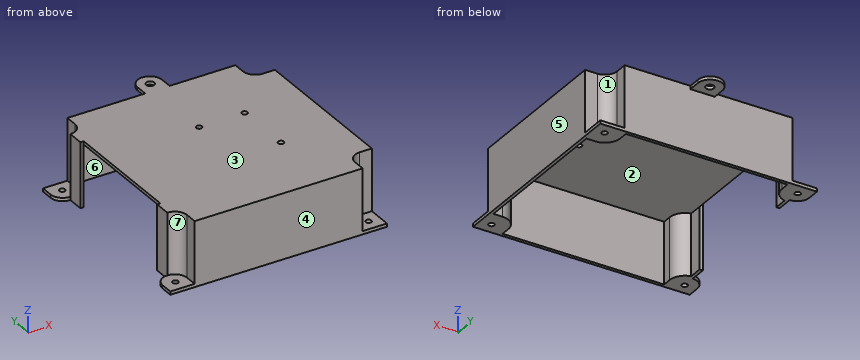
```python
from build123d import *

# Parameters (mm, degrees)
ESQUISSE1_W                = 126
ESQUISSE1_H                = 126
BOSS_EXTRU_1_DEPTH         = 40
ENL_V_MAT_EXTRU_1_DEPTH    = 38
ENL_V_MAT_EXTRU_2_REACH    = 223.428
ESQUISSE4_R                = 1.75
ENL_V_MAT_EXTRU_5_DEPTH    = 38
COQUE1_DEPTH               = 38
BOSS_EXTRU_3_DEPTH         = 2
ENL_V_MAT_EXTRU_6_REACH    = 228.624
ESQUISSE13_R               = 1.75
ENL_V_MAT_EXTRU_7_REACH    = 228.968
ESQUISSE14_R               = 1.75
R_P_TITION_LIN_AIRE1_COUNT = 2
R_P_TITION_LIN_AIRE1_PITCH = 28
ENL_V_MAT_EXTRU_8_REACH    = 228.968
ESQUISSE15_R               = 1.75
ESQUISSE16_W               = 40
ESQUISSE16_H               = 76
ENL_V_MAT_EXTRU_9_DEPTH    = 2
BOSS_EXTRU_4_DEPTH         = 2
ENL_V_MAT_EXTRU_10_REACH   = 239.591
ESQUISSE19_R               = 2.5


# Read off the part's stored shape, not the designer's step: Coque1
with BuildPart() as part:
    # Esquisse1 → Boss.-Extru.1 (new body)
    with BuildSketch(Plane.XY):
        with Locations((-88.440384558, 94.010362694)):
            Rectangle(ESQUISSE1_W, ESQUISSE1_H)
    extrude(amount=BOSS_EXTRU_1_DEPTH)

    # Esquisse2 → Enlèv. mat.-Extru.1 (cut)
    with BuildSketch(Plane.XY.offset(40)):
        with BuildLine():
            Line((-40.440384558, 31.010362694), (-25.440384558, 31.010362694))
            Line((-25.440384558, 31.010362694), (-25.440384558, 46.010362694))
            Line((-25.440384558, 46.010362694), (-32.940384558, 46.010362694))
            ThreePointArc((-32.940384558, 46.010362694), (-38.243685417, 43.813663553), (-40.440384558, 38.510362694))
            Line((-40.440384558, 38.510362694), (-40.440384558, 31.010362694))
        make_face()
    enl_v_mat_extru_1 = extrude(amount=-ENL_V_MAT_EXTRU_1_DEPTH, mode=Mode.SUBTRACT)

    # Esquisse4 → Enlèv. mat.-Extru.2 (cut, up to next)
    with BuildSketch(Plane.XY.offset(2), mode=Mode.PRIVATE) as enl_v_mat_extru_2_sk1:
        with Locations((-32.440384558, 38.010362694)):
            Circle(ESQUISSE4_R)
    enl_v_mat_extru_2_tool1 = extrude(enl_v_mat_extru_2_sk1.sketch, amount=-ENL_V_MAT_EXTRU_2_REACH, mode=Mode.PRIVATE) & part.part
    enl_v_mat_extru_2 = enl_v_mat_extru_2_tool1.solids().sort_by_distance((-32.440385, 38.010363, 2))[0]
    add(enl_v_mat_extru_2, mode=Mode.SUBTRACT)

    # Symétrie1: Enlèv. mat.-Extru.1, Enlèv. mat.-Extru.2 across plane
    add(enl_v_mat_extru_1.mirror(Plane(origin=(0, 94.010362694, 0), x_dir=(0, 0, 1), z_dir=(0, -1, 0))), mode=Mode.SUBTRACT)
    add(enl_v_mat_extru_2.mirror(Plane(origin=(0, 94.010362694, 0), x_dir=(0, 0, 1), z_dir=(0, -1, 0))), mode=Mode.SUBTRACT)

    # Esquisse10 → Enlèv. mat.-Extru.5 (cut)
    with BuildSketch(Plane.XY.offset(40)):
        with BuildLine():
            Line((-151.440384558, 46.010362694), (-151.440384558, 31.010362694))
            Line((-151.440384558, 31.010362694), (-143.940384558, 31.010362694))
            Line((-143.940384558, 31.010362694), (-143.940384558, 38.510362694))
            ThreePointArc((-143.940384558, 38.510362694), (-146.137083699, 43.813663553), (-151.440384558, 46.010362694))
        make_face()
    enl_v_mat_extru_5 = extrude(amount=-ENL_V_MAT_EXTRU_5_DEPTH, mode=Mode.SUBTRACT)

    # Symétrie3: Enlèv. mat.-Extru.5 across plane
    add(enl_v_mat_extru_5.mirror(Plane(origin=(0, 94.010362694, 0), x_dir=(0, 0, 1), z_dir=(0, -1, 0))), mode=Mode.SUBTRACT)

    # Coque1 outline → Coque1 (cut)
    with BuildSketch(Plane.XY):
        with BuildLine():
            Line((-42.440384558, 155.010362694), (-141.940384558, 155.010362694))
            Line((-141.940384558, 155.010362694), (-141.940384558, 149.510362694))
            ThreePointArc((-141.940384558, 149.510362694), (-144.049511808, 143.541694501), (-149.440384558, 140.223274884))
            Line((-149.440384558, 140.223274884), (-149.440384558, 47.797450505))
            ThreePointArc((-149.440384558, 47.797450505), (-144.049511808, 44.479030887), (-141.940384558, 38.510362694))
            Line((-141.940384558, 38.510362694), (-141.940384558, 33.010362694))
            Line((-141.940384558, 33.010362694), (-42.440384558, 33.010362694))
            Line((-42.440384558, 33.010362694), (-42.440384558, 38.510362694))
            ThreePointArc((-42.440384558, 38.510362694), (-39.657898979, 45.227877116), (-32.940384558, 48.010362694))
            Line((-32.940384558, 48.010362694), (-27.440384558, 48.010362694))
            Line((-27.440384558, 48.010362694), (-27.440384558, 140.010362694))
            Line((-27.440384558, 140.010362694), (-32.940384558, 140.010362694))
            ThreePointArc((-32.940384558, 140.010362694), (-39.657898979, 142.792848273), (-42.440384558, 149.510362694))
            Line((-42.440384558, 149.510362694), (-42.440384558, 155.010362694))
        make_face()
    extrude(amount=COQUE1_DEPTH, mode=Mode.SUBTRACT)

    # Esquisse12 → Boss.-Extru.3 (add)
    with BuildSketch(Plane.XY.offset(2)):
        with BuildLine():
            Line((-158.940384558, 31.010362694), (-158.940384558, 38.510362694))
            ThreePointArc((-158.940384558, 38.510362694), (-156.743685417, 43.813663553), (-151.440384558, 46.010362694))
            Line((-151.440384558, 46.010362694), (-151.440384558, 31.010362694))
            Line((-151.440384558, 31.010362694), (-158.940384558, 31.010362694))
        make_face()
    boss_extru_3 = extrude(amount=-BOSS_EXTRU_3_DEPTH)

    # Esquisse13 → Enlèv. mat.-Extru.6 (cut, up to next)
    with BuildSketch(Plane.XY.offset(2), mode=Mode.PRIVATE) as enl_v_mat_extru_6_sk1:
        with Locations((-151.440384558, 38.010362694)):
            Circle(ESQUISSE13_R)
    enl_v_mat_extru_6_tool1 = extrude(enl_v_mat_extru_6_sk1.sketch, amount=-ENL_V_MAT_EXTRU_6_REACH, mode=Mode.PRIVATE) & part.part
    enl_v_mat_extru_6 = enl_v_mat_extru_6_tool1.solids().sort_by_distance((-151.440385, 38.010363, 2))[0]
    add(enl_v_mat_extru_6, mode=Mode.SUBTRACT)

    # Symétrie5: Boss.-Extru.3, Enlèv. mat.-Extru.6 across plane
    add(boss_extru_3.mirror(Plane(origin=(0, 94.010362694, 0), x_dir=(0, 0, 1), z_dir=(0, -1, 0))))
    add(enl_v_mat_extru_6.mirror(Plane(origin=(0, 94.010362694, 0), x_dir=(0, 0, 1), z_dir=(0, -1, 0))), mode=Mode.SUBTRACT)

    # Esquisse14 → Enlèv. mat.-Extru.7 (cut, up to next)
    with BuildSketch(Plane.XY.offset(40), mode=Mode.PRIVATE) as enl_v_mat_extru_7_sk1:
        with Locations((-90.440384558, 112.510362694)):
            Circle(ESQUISSE14_R)
    enl_v_mat_extru_7_tool1 = extrude(enl_v_mat_extru_7_sk1.sketch, amount=-ENL_V_MAT_EXTRU_7_REACH, mode=Mode.PRIVATE) & part.part
    enl_v_mat_extru_7 = enl_v_mat_extru_7_tool1.solids().sort_by_distance((-90.440385, 112.510363, 40))[0]
    add(enl_v_mat_extru_7, mode=Mode.SUBTRACT)

    # Répétition linéaire1: Enlèv. mat.-Extru.7 ×2
    with Locations(*[(i * R_P_TITION_LIN_AIRE1_PITCH, 0, 0) for i in range(1, R_P_TITION_LIN_AIRE1_COUNT)]):
        add(enl_v_mat_extru_7, mode=Mode.SUBTRACT)

    # Esquisse15 → Enlèv. mat.-Extru.8 (cut, up to next)
    with BuildSketch(Plane.XY.offset(40), mode=Mode.PRIVATE) as enl_v_mat_extru_8_sk1:
        with Locations((-62.440384558, 76.510362694)):
            Circle(ESQUISSE15_R)
    enl_v_mat_extru_8_tool1 = extrude(enl_v_mat_extru_8_sk1.sketch, amount=-ENL_V_MAT_EXTRU_8_REACH, mode=Mode.PRIVATE) & part.part
    add(enl_v_mat_extru_8_tool1.solids().sort_by_distance((-62.440385, 76.510363, 40))[0], mode=Mode.SUBTRACT)

    # Esquisse16 → Enlèv. mat.-Extru.9 (cut)
    with BuildSketch(Plane.ZY.offset(151.440384558)):
        with Locations((20, 94.010362694)):
            Rectangle(ESQUISSE16_W, ESQUISSE16_H)
    extrude(amount=-ENL_V_MAT_EXTRU_9_DEPTH, mode=Mode.SUBTRACT)

    # Esquisse17 → Boss.-Extru.4 (add)
    with BuildSketch(Plane.XY.offset(40)):
        with BuildLine():
            Line((-95.940384558, 157.010362694), (-80.940384558, 157.010362694))
            Line((-80.940384558, 157.010362694), (-80.940384558, 164.510362694))
            ThreePointArc((-80.940384558, 164.510362694), (-88.440384558, 172.010362694), (-95.940384558, 164.510362694))
            Line((-95.940384558, 164.510362694), (-95.940384558, 157.010362694))
        make_face()
    extrude(amount=-BOSS_EXTRU_4_DEPTH)

    # Esquisse19 → Enlèv. mat.-Extru.10 (cut, up to next)
    with BuildSketch(Plane.XY.offset(40), mode=Mode.PRIVATE) as enl_v_mat_extru_10_sk1:
        with Locations((-88.440384558, 164.260362694)):
            Circle(ESQUISSE19_R)
    enl_v_mat_extru_10_tool1 = extrude(enl_v_mat_extru_10_sk1.sketch, amount=-ENL_V_MAT_EXTRU_10_REACH, mode=Mode.PRIVATE) & part.part
    add(enl_v_mat_extru_10_tool1.solids().sort_by_distance((-88.440385, 164.260363, 40))[0], mode=Mode.SUBTRACT)


solid = part.part
```
Model file for the job. Use its own axes, mm. Face numbers are marked on the shaded views. A direction names the side the tool comes from. Coordinates: 2 decimals unless noted, no trailing zeros. Write each loop counter-clockwise with the first axis right and the second up, starting at its lowest first coordinate (ties: lowest second). Pieces come first, ordered by that corner, then holes. Notation, with made-up numbers: (60.25, 9) - (75.25, 9) arc R24 ccw to (75.25, 38) - close; hole circle Ø9 at (65.25, -23.75). An arc over 180 degrees is marked (long way). One line per item, written item: value. Start each with the question number.
1. Slice it at A-A (y = 95). Write the cut outline in (x, z).
2. Mould opens along Y. For the marked faces 1, 2, 3 and 4 say: released by +Y, released by -Y, zero draft, split by the parting line, or undercut.
3. Tool access for the marked faces 5, 6 and 7: list every direction of +Z, -Z, +X, -X, +Y, -Y with a clear straight run to the whole face (end or side of a thin tool).
4. Probe line 1 (Y direction, x = -32, z = 15); line 2 (Y direction, x = -124, z = 16); line 3 (X direction, y = 69.5, z = 26). List the from-to ranges inside material, lowest first. Write a range as from..to.
5. Flat gauge pins, fed straight in: pin 1 (4.5 mm diameter, centred on y = 152, z = 13, fed in from -X); pin 2 (20 mm diameter, centred on x = -71.5, z = 12, fed in from +Y); pin 3 (1.6 mm diameter, centred on y = 162, z = 39, fed in from +X); pin 4 (3 mm diameter, centred on x = -32.44, y = 150.01, fed in from +Z). Where does each tip first touch, or does it go through?
6. Slice it at B-B (x = -75.5). Write the cut outline in (y, z), plus the area to 3 significant figures.
7. Slice it at D-D (x = -36). Write the cut outline in (y, z).
Answers below:
1. outline: (-149.44, 38) - (-27.44, 38) - (-27.44, 0) - (-25.44, 0) - (-25.44, 40) - (-149.44, 40) - close
2. face 1: released by +Y
2. face 2: undercut
2. face 3: zero draft
2. face 4: released by -Y
3. face 5: +Z, -Z, +X, +Y, -Y
3. face 6: -Z
3. face 7: +Z, -X, -Y
4. line 1: y = 46.01..48.01, 140.01..142.01
4. line 2: y = 31.01..33.01, 155.01..157.01
4. line 3: x = -27.44..-25.44
5. pin 1: stops at x = -143.94
5. pin 2: stops at y = 157.01
5. pin 3: stops at x = -80.94
5. pin 4: passes through
6. outline: (31.01, 0) - (33.01, 0) - (33.01, 38) - (155.01, 38) - (155.01, 0) - (157.01, 0) - (157.01, 40) - (31.01, 40) - close
6. area: 404 mm^2
7. outline: (31.01, 0) - (47.5, 0) - (47.5, 38) - (140.52, 38) - (140.52, 0) - (157.01, 0) - (157.01, 2) - (142.66, 2) - (142.66, 40) - (45.36, 40) - (45.36, 2) - (31.01, 2) - close
